from build123d import *

# Parameters (mm, degrees)
SKETCH1_W           = 30.4
SKETCH1_H           = 3.2
BOSS_EXTRUDE1_DEPTH = 17.6
SKETCH2_R           = 1.5
CUT_EXTRUDE1_DEPTH  = 16
SKETCH3_R           = 1.075
CUT_EXTRUDE2_DEPTH  = 16
SKETCH4_W           = 22.4
SKETCH4_H           = 3.2
BOSS_EXTRUDE2_DEPTH = 12.8
SKETCH5_R           = 1.075
CUT_EXTRUDE3_DEPTH  = 16
FILLET1_R           = 10
FILLET2_R           = 4
FILLET3_R           = 2


with BuildPart() as part:
    # Sketch1 → Boss-Extrude1 (new body)
    with BuildSketch(Plane(origin=(0, 0, 0), x_dir=(1, 0, 0), z_dir=(0, 1, 0))):
        with Locations((15.2, -1.6)):
            Rectangle(SKETCH1_W, SKETCH1_H)
    extrude(amount=BOSS_EXTRUDE1_DEPTH)

    # Sketch2 → Cut-Extrude1 (cut)
    with BuildSketch(Plane.XY.offset(3.2)):
        with Locations((23.2, 6.4)):
            Circle(SKETCH2_R)
        with Locations((7.2, 6.4)):
            Circle(SKETCH2_R)
    extrude(amount=-CUT_EXTRUDE1_DEPTH, mode=Mode.SUBTRACT)

    # Sketch3 → Cut-Extrude2 (cut)
    with BuildSketch(Plane(origin=(0, 0, 0), x_dir=(-1, 0, 0), z_dir=(0, 0, -1))):
        with Locations((-27.2, 12.8)):
            Circle(SKETCH3_R)
        with Locations((-3.2, 12.8)):
            Circle(SKETCH3_R)
    extrude(amount=-CUT_EXTRUDE2_DEPTH, mode=Mode.SUBTRACT)

    # Sketch4 → Boss-Extrude2 (add)
    with BuildSketch(Plane(origin=(0, 17.6, 0), x_dir=(1, 0, 0), z_dir=(0, 1, 0))):
        with Locations((15.2, -1.6)):
            Rectangle(SKETCH4_W, SKETCH4_H)
    extrude(amount=BOSS_EXTRUDE2_DEPTH)

    # Sketch5 → Cut-Extrude3 (cut)
    with BuildSketch(Plane.XY.offset(3.2)):
        with Locations((12, 24)):
            Circle(SKETCH5_R)
    extrude(amount=-CUT_EXTRUDE3_DEPTH, mode=Mode.SUBTRACT)

    # Fillet1
    fillet1_edges = [part.edges().sort_by_distance(p)[0] for p in [
        (4, 30.4, 1.6),
        (26.4, 30.4, 1.6),
    ]]
    fillet(fillet1_edges, radius=FILLET1_R)

    # Fillet2
    fillet2_edges = [part.edges().sort_by_distance(p)[0] for p in [
        (30.4, 17.6, 1.6),
        (0, 17.6, 1.6),
    ]]
    fillet(fillet2_edges, radius=FILLET2_R - 0.0001)  # a hair under: the kernel refuses the full size

    # Fillet3
    fillet3_edges = [part.edges().sort_by_distance(p)[0] for p in [
        (4, 17.6, 1.6),
        (26.4, 17.6, 1.6),
    ]]
    fillet(fillet3_edges, radius=FILLET3_R)


solid = part.part
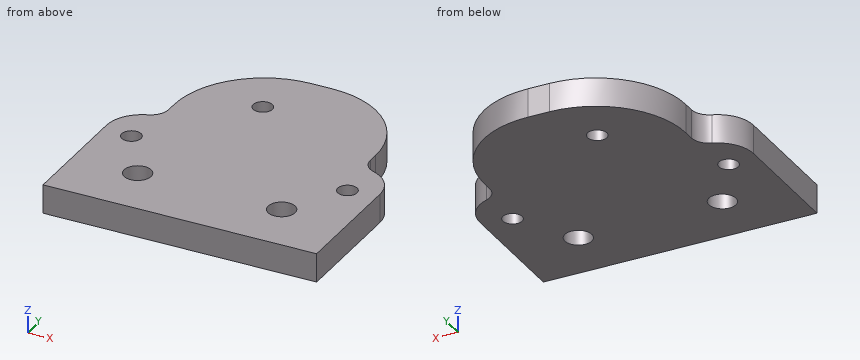
Source: CAD feature listing. Evaluate the final solid. Frame: model axes, mm. Round coordinates to 2 decimals unless told otherwise and drop trailing zeros. Order: outer loops, then holes, each group sorted by start corner. A loop starts at its lowest first (then second) coordinate and runs counter-clockwise, first axis right, second up. Notation, with made-up numbers: (13.5, -23) -> (19.5, -23) arc R25 ccw to (19.5, 12) -> close; hole circle Ø3 at (39.5, -26). An arc over 180 degrees is marked (long way). Answer as CSV lines item,"result".
Item 1: Line query: L1, parallel to X at y = 6.5, z = 1.4; L2, parallel to X at y = 12.5, z = 1.65; L3, parallel to Y at x = 23.2, z = 1.95. Output: solid intervals per line, ascending.
A:
L1,"0 to 5.7, 8.7 to 21.7, 24.7 to 30.4"
L2,"0 to 2.17, 4.23 to 26.17, 28.23 to 30.4"
L3,"0 to 4.9, 7.9 to 27.73"
Item 2: Section D-D, the plane z = 2. Count the separate pieces of the cut face and the enclosed holes in it, plus the area to 3 significant figures.
A:
separate pieces,"1"
enclosed holes,"5"
area,"748 mm²"
Item 3: Pin query (flat end, axial travel): pin 1 Ø1.5 at (x, z) = (19.5, 1) entering from +Y; pin 2 Ø0.9 at (y, z) = (19.5, 2) entering from +X; pin 3 Ø1.3 at (y, z) = (19.5, 2) entering from -X. Return the tip coordinate at first contact, or that it passes through.
A:
pin 1,"y = 30.12"
pin 2,"x = 26.41"
pin 3,"x = 3.96"
Item 4: Section A-A, the plane y = 5.5. Return loops of the section in (x, z).
A:
outline,"(0, 0) -> (6, 0) -> (6, 3.2) -> (0, 3.2) -> close; (8.4, 0) -> (22, 0) -> (22, 3.2) -> (8.4, 3.2) -> close; (24.4, 0) -> (30.4, 0) -> (30.4, 3.2) -> (24.4, 3.2) -> close"
Item 5: Section B-B, the plane x = 7. Return loops of the section in (y, z).
A:
outline,"(0, 0) -> (4.91, 0) -> (4.91, 3.2) -> (0, 3.2) -> close; (7.89, 0) -> (27.54, 0) -> (27.54, 3.2) -> (7.89, 3.2) -> close"
Item 6: Section C-C, the plane y = 24. Return loops of the section in (x, z) (3 decimals).
A:
outline,"(4.67, 0) -> (10.925, 0) -> (10.925, 3.2) -> (4.67, 3.2) -> close; (13.075, 0) -> (25.73, 0) -> (25.73, 3.2) -> (13.075, 3.2) -> close"
